CAD build for the part. Positions are in the model's coordinates, mm. Coordinates: 2 decimals unless noted, no trailing zeros. Loops run counter-clockwise (first coordinate to the right, second up) from the corner with the lowest first, then second, coordinate; pieces in that order, holes last. Notation, with made-up numbers: (48.5, 16.5) - (60.5, 16.5) arc R22 ccw to (60.5, 53.5) - close; hole circle Ø4 at (80.5, 48). An arc over 180 degrees is marked (long way). Put each result on its own line as item: value.
```python
from build123d import *

# Parameters (mm, degrees)
BOSS_EXTRUDE6_DEPTH = 4


with BuildPart() as part:
    # Sketch20 → Boss-Extrude6 (new body)
    with BuildSketch(Plane.XY):
        with BuildLine():
            Line((36.624785701, -24.701414589), (17.902939914, -56.058435219))
            Line((17.902939914, -56.058435219), (31.951161852, -297.999999834))
            Line((31.951161852, -297.999999834), (-16.59209867, -298.052484048))
            Line((-16.59209867, -298.052484048), (-16.59209867, -7.784403475))
            Line((-16.59209867, -7.784403475), (-11.309666824, -6.069762931))
            Line((-11.309666824, -6.069762931), (17.938518552, -15.571491158))
            Line((17.938518552, -15.571491158), (24.592593053, -11.700714256))
            ThreePointArc((24.592593053, -11.700714256), (35.424716451, -13.743814885), (36.624785701, -24.701414589))
        make_face()
        with BuildLine():
            Line((-6.6408348, -18.644095931), (-6.337063012, -19.478702059))
            ThreePointArc((-6.337063012, -19.478702059), (-5.755598413, -20.391418654), (-4.842881819, -20.972883253))
            Line((-4.842881819, -20.972883253), (9.594949642, -26.227824152))
            ThreePointArc((9.594949642, -26.227824152), (11.883941091, -25.92647271), (12.95, -23.8785926))
            Line((12.95, -23.8785926), (12.95, -18.302075788))
            ThreePointArc((12.95, -18.302075788), (12.657106781, -17.594969007), (11.95, -17.302075788))
            Line((11.95, -17.302075788), (-5.701142179, -17.302075788))
            ThreePointArc((-5.701142179, -17.302075788), (-6.520294224, -17.728499352), (-6.6408348, -18.644095931))
        make_face(mode=Mode.SUBTRACT)
        with BuildLine():
            Line((-1.8643328, -31.767427321), (3.165925841, -45.587949351))
            ThreePointArc((3.165925841, -45.587949351), (4.062910493, -46.756922509), (5.468172762, -47.2))
            Line((5.468172762, -47.2), (10.5, -47.2))
            ThreePointArc((10.5, -47.2), (12.232411614, -46.482411614), (12.95, -44.75))
            Line((12.95, -44.75), (12.95, -34.591777725))
            ThreePointArc((12.95, -34.591777725), (12.506922509, -33.186515456), (11.337949351, -32.289530804))
            Line((11.337949351, -32.289530804), (1.275863472, -28.627231049))
            ThreePointArc((1.275863472, -28.627231049), (-1.294497493, -29.197066356), (-1.8643328, -31.767427321))
        make_face(mode=Mode.SUBTRACT)
    extrude(amount=BOSS_EXTRUDE6_DEPTH)


solid = part.part
```
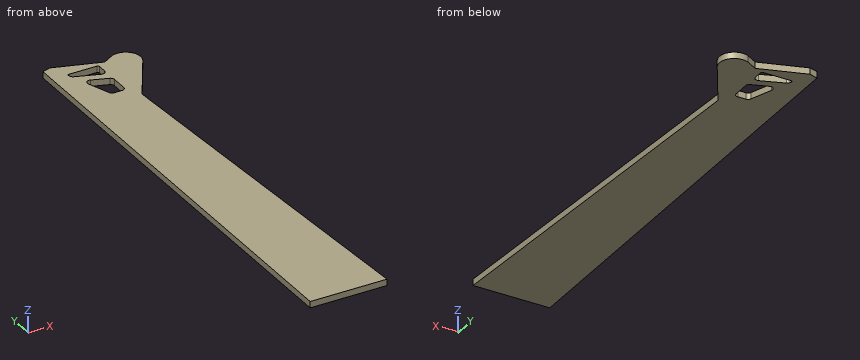
Q1. Slice it at B-B, the plane y = -151.5. Give the cut face in (x, z).
Determined:
outline: (-16.59, 0) - (23.44, 0) - (23.44, 4) - (-16.59, 4) - close
Q2. Slice it at A-A, the plane z = 3.2. Give the cut face in (x, y).
Determined:
outline: (-16.59, -298.05) - (31.95, -298) - (17.9, -56.06) - (36.62, -24.7) arc R9.26 ccw to (24.59, -11.7) - (17.94, -15.57) - (-11.31, -6.07) - (-16.59, -7.78) - close; hole (-6.64, -18.64) - (-6.34, -19.48) arc R2.5 ccw to (-4.84, -20.97) - (9.59, -26.23) arc R2.5 ccw to (12.95, -23.88) - (12.95, -18.3) arc R1 ccw to (11.95, -17.3) - (-5.7, -17.3) arc R1 ccw to start; hole (-1.86, -31.77) - (3.17, -45.59) arc R2.45 ccw to (5.47, -47.2) - (10.5, -47.2) arc R2.45 ccw to (12.95, -44.75) - (12.95, -34.59) arc R2.45 ccw to (11.34, -32.29) - (1.28, -28.63) arc R2.45 ccw to start
Q3. Pin check, flat tips, straight feed: pin 1 Ø1 at (x, z) = (8.5, 1.5) entering from +Y; pin 2 Ø8 at (x, y) = (25.5, -127.5) entering from -Z; pin 3 Ø2 at (x, z) = (6.5, 1) entering from -Y; pin 4 Ø1 at (y, z) = (-171.5, 3) entering from +X. Stop position of each tip, or through.
Determined:
pin 1: y = -12.34
pin 2: z = 0
pin 3: y = -298.03
pin 4: x = 24.64
Q4. Slice it at C-C, the plane y = -117. Give the cut face in (x, z).
Determined:
outline: (-16.59, 0) - (21.44, 0) - (21.44, 4) - (-16.59, 4) - close
Q5. Wall check: L1, parallel to Y at x = 11, z = 1.05; L2, parallel to X at y = -41.5, z = 2; L3, parallel to Y at x = -5.5, z = 3.6. Give the ranges that are in metal, low to high. Write a range as from..to.
Determined:
L1: -298.02..-47.15, -32.17..-26.32, -17.3..-13.32
L2: -16.59..1.68, 12.95..26.6
L3: -298.04..-20.61, -17.3..-7.96
